Input: part model. Units: mm. Frame: model coordinates. Coordinates: 2 decimals unless noted, no trailing zeros. Write each loop counter-clockwise with the first axis right and the second up, starting at its lowest first coordinate (ties: lowest second). Pieces come first, ordered by that corner, then holes. Notation, with made-up numbers: (87, 4.25) - (129, 4.25) arc R7 ccw to (129, 10.25) - close; hole circle Ø1 at (81, -38.5). An arc over 180 degrees is marked (long way). Put each result on its own line as item: value. Start each with the question number.
1. Pin query (flat end, axial travel): pin 1 (1.5 mm diameter, centred on y = 1, z = 5, fed in from +X); pin 2 (2 mm diameter, centred on x = 5.5, z = 1, fed in from -Y). Return the tip coordinate at first contact, or that it passes through.
2. Pull-direction query (Y, two-part tool) for faces 1 (the flat face through (0, -6.5, 3)), 2 (the conical face through (-3.621, 5.685, 0.139)), 3 (the cylindrical face through (-2.539, -1.947, 3.436)); classes: released by +Y, released by -Y, zero draft, split by the parting line, or undercut.
3. Line query: line 1 (X direction, y = 0.25, z = 2.25); line 2 (X direction, y = -2, z = 2.5); line 3 (Y direction, x = 1.5, z = 5.5). Output: solid intervals per line, ascending.
4. Cut plane A-A, the plane z = 4.25. Return loops of the section in (x, y).
from build123d import *

# Parameters (mm, degrees)
BASE_EXTRUSION_DEPTH    = 6.8
ESQUISSE4_R             = 3.2
ENL_V_MAT_EXTRU_1_DEPTH = 12.840021115
CHANFREIN1_SIZE         = 0.8


with BuildPart() as part:
    # Esquisse1 → Base-Extrusion (new body)
    with BuildSketch(Plane.XY):
        Polygon((-7.19, 0), (-4.116549171, 6.5), (4.116549171, 6.5), (7.19, 0), (4.116549171, -6.5), (-4.116549171, -6.5), align=None)
    extrude(amount=BASE_EXTRUSION_DEPTH)

    # Esquisse3 → Enlever de la matière-Révolution1 (revolve, cut)
    with BuildSketch(Plane(origin=(0, 0, 0), x_dir=(0, 0, -1), z_dir=(1, 0, 0)), mode=Mode.PRIVATE) as enlever_de_la_mati_re_r_volution1_sk:
        Polygon((-6.8, 6.5), (-3.4, 12.388972746), (0, 6.5), (2.598076211, 8), (-3.4, 18.388972746), (-9.398076211, 8), align=None)
    revolve(enlever_de_la_mati_re_r_volution1_sk.sketch.rotate(Axis((0, 0, 8.495961775), (0, 0, -1)), 90), axis=Axis((0, 0, 8.495961775), (0, 0, -1)), mode=Mode.SUBTRACT)

    # Esquisse4 → Enlèv. mat.-Extru.1 (cut, through all)
    with BuildSketch(Plane.XY.offset(6.8)):
        Circle(ESQUISSE4_R)
    extrude(amount=-ENL_V_MAT_EXTRU_1_DEPTH, mode=Mode.SUBTRACT)

    # Chanfrein1
    chanfrein1_edges = [part.edges().sort_by_distance(p)[0] for p in [
        (-3.2, 0, 0),
        (-3.2, 0, 6.8),
    ]]
    chamfer(chanfrein1_edges, length=CHANFREIN1_SIZE)


solid = part.part
Report:
1. pin 1: stops at x = 7.07
1. pin 2: stops at y = -5.69
2. face 1: released by -Y
2. face 2: released by +Y
2. face 3: undercut
3. line 1: x = -7.07 to -3.19, 3.19 to 7.07
3. line 2: x = -6.24 to -2.5, 2.5 to 6.24
3. line 3: y = -6.5 to -2.83, 2.83 to 6.5
4. outline: (-7.19, 0) - (-4.12, -6.5) - (4.12, -6.5) - (7.19, 0) - (4.12, 6.5) - (-4.12, 6.5) - close; hole circle Ø6.4 at (0, 0)
